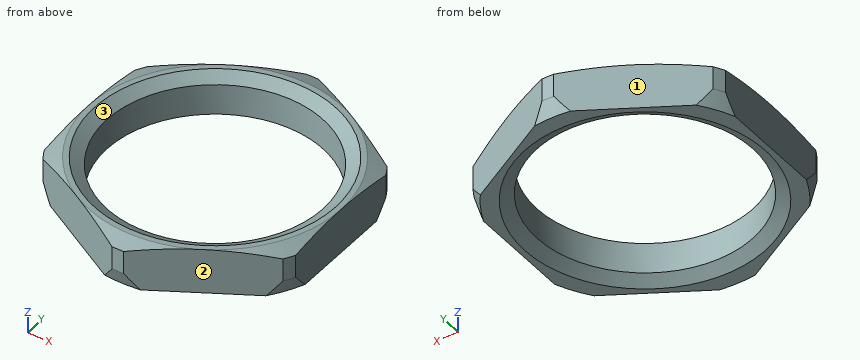
from build123d import *

# Parameters (mm, degrees)
BOSS_EXTRUDE1_DEPTH   = 2.5
HOLE1_D               = 12
HOLE1_DEPTH           = 2.5
CHAMFER1_SIZE         = 0.9
CHAMFER1_SIZE2        = 0.327573212
CHAMFER1_PART_2_SIZE  = 0.9
CHAMFER1_PART_2_SIZE2 = 0.327573212
CHAMFER1_PART_3_SIZE  = 0.9
CHAMFER1_PART_3_SIZE2 = 0.327573212
CHAMFER1_PART_4_SIZE  = 0.9
CHAMFER1_PART_4_SIZE2 = 0.327573212
CHAMFER1_PART_5_SIZE  = 0.9
CHAMFER1_PART_5_SIZE2 = 0.327573212
CHAMFER1_PART_6_SIZE  = 0.9
CHAMFER1_PART_6_SIZE2 = 0.327573212
CHAMFER1_PART_7_SIZE  = 0.9
CHAMFER1_PART_7_SIZE2 = 0.327573212
CHAMFER2_SIZE         = 0.692820323
CHAMFER2_SIZE2        = 0.400000001
CHAMFER3_SIZE         = 0.692820323
CHAMFER3_SIZE2        = 0.400000001


with BuildPart() as part:
    # Sketch1 → Boss-Extrude1 (new body)
    with BuildSketch(Plane(origin=(0, 0, 6), x_dir=(-1, 0, 0), z_dir=(0, 0, -1))):
        with BuildLine():
            Line((-7, 3.661966685), (-7, -3.661966685))
            ThreePointArc((-7, -3.661966685), (-6.84160069, -3.95), (-6.671356177, -4.231194484))
            Line((-6.671356177, -4.231194484), (-0.328643823, -7.893161169))
            ThreePointArc((-0.328643823, -7.893161169), (0, -7.9), (0.328643823, -7.893161169))
            Line((0.328643823, -7.893161169), (6.671356177, -4.231194484))
            ThreePointArc((6.671356177, -4.231194484), (6.84160069, -3.95), (7, -3.661966685))
            Line((7, -3.661966685), (7, 3.661966685))
            ThreePointArc((7, 3.661966685), (6.84160069, 3.95), (6.671356177, 4.231194484))
            Line((6.671356177, 4.231194484), (0.328643823, 7.893161169))
            ThreePointArc((0.328643823, 7.893161169), (0, 7.9), (-0.328643823, 7.893161169))
            Line((-0.328643823, 7.893161169), (-6.671356177, 4.231194484))
            ThreePointArc((-6.671356177, 4.231194484), (-6.84160069, 3.95), (-7, 3.661966685))
        make_face()
    extrude(amount=-BOSS_EXTRUDE1_DEPTH)

    # Hole1
    with Locations(Plane(origin=(0, 0, 6), x_dir=(-1, 0, 0), z_dir=(0, 0, -1))):
        with Locations((0, 0)):
            Hole(HOLE1_D / 2, depth=HOLE1_DEPTH)

    # Chamfer1
    chamfer1_edges = [part.edges().sort_by_distance(p)[0] for p in [
        (0, -7.9, 8.5),
        (-6.84160069, 3.95, 8.5),
        (6.84160069, 3.95, 8.5),
        (6.84160069, -3.95, 8.5),
        (0, 7.9, 8.5),
        (-6.84160069, -3.95, 8.5),
    ]]
    chamfer1_side = [part.faces().sort_by_distance(p)[0] for p in [
        (3.394449064, 5.879358243, 8.5),
    ]]
    chamfer(chamfer1_edges, length=CHAMFER1_SIZE, length2=CHAMFER1_SIZE2, reference=chamfer1_side[0])

    # Chamfer1 part 2
    chamfer1_part_2_edges = [part.edges().sort_by_distance(p)[0] for p in [
        (6.84160069, 3.95, 6),
    ]]
    chamfer1_part_2_side = [part.faces().sort_by_distance(p)[0] for p in [
        (6.84160069, 3.95, 7.25),
    ]]
    chamfer(chamfer1_part_2_edges, length=CHAMFER1_PART_2_SIZE, length2=CHAMFER1_PART_2_SIZE2, reference=chamfer1_part_2_side[0])

    # Chamfer1 part 3
    chamfer1_part_3_edges = [part.edges().sort_by_distance(p)[0] for p in [
        (0, 7.9, 6),
    ]]
    chamfer1_part_3_side = [part.faces().sort_by_distance(p)[0] for p in [
        (0, 7.9, 7.25),
    ]]
    chamfer(chamfer1_part_3_edges, length=CHAMFER1_PART_3_SIZE, length2=CHAMFER1_PART_3_SIZE2, reference=chamfer1_part_3_side[0])

    # Chamfer1 part 4
    chamfer1_part_4_edges = [part.edges().sort_by_distance(p)[0] for p in [
        (-6.84160069, 3.95, 6),
    ]]
    chamfer1_part_4_side = [part.faces().sort_by_distance(p)[0] for p in [
        (-6.84160069, 3.95, 7.25),
    ]]
    chamfer(chamfer1_part_4_edges, length=CHAMFER1_PART_4_SIZE, length2=CHAMFER1_PART_4_SIZE2, reference=chamfer1_part_4_side[0])

    # Chamfer1 part 5
    chamfer1_part_5_edges = [part.edges().sort_by_distance(p)[0] for p in [
        (-6.84160069, -3.95, 6),
    ]]
    chamfer1_part_5_side = [part.faces().sort_by_distance(p)[0] for p in [
        (-6.84160069, -3.95, 7.25),
    ]]
    chamfer(chamfer1_part_5_edges, length=CHAMFER1_PART_5_SIZE, length2=CHAMFER1_PART_5_SIZE2, reference=chamfer1_part_5_side[0])

    # Chamfer1 part 6
    chamfer1_part_6_edges = [part.edges().sort_by_distance(p)[0] for p in [
        (0, -7.9, 6),
    ]]
    chamfer1_part_6_side = [part.faces().sort_by_distance(p)[0] for p in [
        (0, -7.9, 7.25),
    ]]
    chamfer(chamfer1_part_6_edges, length=CHAMFER1_PART_6_SIZE, length2=CHAMFER1_PART_6_SIZE2, reference=chamfer1_part_6_side[0])

    # Chamfer1 part 7
    chamfer1_part_7_edges = [part.edges().sort_by_distance(p)[0] for p in [
        (6.84160069, -3.95, 6),
    ]]
    chamfer1_part_7_side = [part.faces().sort_by_distance(p)[0] for p in [
        (6.84160069, -3.95, 7.25),
    ]]
    chamfer(chamfer1_part_7_edges, length=CHAMFER1_PART_7_SIZE, length2=CHAMFER1_PART_7_SIZE2, reference=chamfer1_part_7_side[0])

    # Chamfer2
    chamfer2_edges = [part.edges().sort_by_distance(p)[0] for p in [
        (-6, 0, 6),
    ]]
    chamfer2_side = [part.faces().sort_by_distance(p)[0] for p in [
        (3.396877913, -5.883565133, 6),
    ]]
    chamfer(chamfer2_edges, length=CHAMFER2_SIZE, length2=CHAMFER2_SIZE2, reference=chamfer2_side[0])

    # Chamfer3
    chamfer3_edges = [part.edges().sort_by_distance(p)[0] for p in [
        (-6, 0, 8.5),
    ]]
    chamfer3_side = [part.faces().sort_by_distance(p)[0] for p in [
        (3.401005054, 5.890713542, 8.5),
    ]]
    chamfer(chamfer3_edges, length=CHAMFER3_SIZE, length2=CHAMFER3_SIZE2, reference=chamfer3_side[0])


solid = part.part
Verification items for the finished model (mm, model axes). Face numbers are marked on the shaded views. Give positions to 0.01 mm unless a question says otherwise; leave off trailing zeros. Loops run counter-clockwise (first coordinate to the right, second up) from the corner with the lowest first, then second, coordinate; pieces in that order, holes last.
1. Material ranges on probe 1 along Y at (x, z) = (0, 7.55); probe 2 along X at (y, z) = (-1, 6.75); probe 3 along Y at (x, z) = (-5.25, 7.8), recorded low to high.
Derived:
probe 1: y = -7.9 to -6, 6 to 7.9
probe 2: x = -7 to -5.92, 5.92 to 7
probe 3: y = -5.05 to -2.9, 2.9 to 5.05
2. Release check for a two-part mould opening along X. For the marked faces 1, 2 and 3 record: +X half, -X half, draft (parallel to the pull), parting line (faces both ways), or undercut.
Derived:
face 1: -X half
face 2: +X half
face 3: undercut
3. Go/stop test with flat-tipped pins: P1, Ø1, axis at x = -5.5, z = 7.5, coming from the +Y side; P2, Ø1, axis at x = -1, z = 6.5, coming from the +Y side; P3, Ø1, axis at x = -3.5, y = 4.5, coming from the +Z side. Record where each tip stops, or that it passes through.
Derived:
P1: stops at y = 5.2
P2: stops at y = 7.78
P3: stops at z = 8.22
4. Cross-section at A-A on z = 7.9. Record the cut outline in (x, y), and give its area (3 significant figures).
Derived:
outline: (-7, -3.66) arc R7.9 ccw to (-6.67, -4.23) - (-0.33, -7.89) arc R7.9 ccw to (0.33, -7.89) - (6.67, -4.23) arc R7.9 ccw to (7, -3.66) - (7, 3.66) arc R7.9 ccw to (6.67, 4.23) - (0.33, 7.89) arc R7.9 ccw to (-0.33, 7.89) - (-6.67, 4.23) arc R7.9 ccw to (-7, 3.66) - close; hole circle Ø12 at (0, 0)
area: 56.3 mm2
5. Cross-section at B-B on x = 0. Record the cut outline in (y, z), and give its area (3 significant figures).
Derived:
outline: (-7.9, 6.9) - (-7.57, 6) - (-6.69, 6) - (-6, 6.4) - (-6, 8.1) - (-6.69, 8.5) - (-7, 8.5) - (-7.9, 8.17) - close; (6, 6.4) - (6.69, 6) - (7.57, 6) - (7.9, 6.9) - (7.9, 8.17) - (7, 8.5) - (6.69, 8.5) - (6, 8.1) - close
area: 8.36 mm2
